Part model, mm, in its own coordinate system. Face numbers are marked on the shaded views. A direction names the side the tool comes from. Coordinates: 2 decimals unless noted, no trailing zeros. Loops run counter-clockwise (first coordinate to the right, second up) from the corner with the lowest first, then second, coordinate; pieces in that order, holes last.
Solid Edge part; units mm, degrees
sketch "Sketch1" plane through (0, 0, 0) normal (0, -1, 0) x (1, 0, 0)
  circle A0 centre (80.5127, 55.3877) radius 22.5
extrude "ExtrudedProtrusion_1" add sketch "Sketch1" against normal blind 10
sketch "Sketch2" plane through (63.9305, 0, 41.9251) normal (0, -1, 0) x (1, 0, 0)
  line L0 (18.5822, 5.9759) -> (18.5822, 0.9759)
  arc A0 (18.5822, 0.9759) -> (14.5822, 0.9759) centre (16.5822, 0.9759) cw
  line L1 (14.5822, 0.9759) -> (14.5822, 5.9759)
  arc A1 (14.5822, 5.9759) -> (9.5822, 10.9759) centre (9.5822, 5.9759) ccw
  line L2 (9.5822, 10.9759) -> (4.5822, 10.9759)
  arc A2 (4.5822, 10.9759) -> (4.5822, 14.9759) centre (4.5822, 12.9759) cw
  line L3 (4.5822, 14.9759) -> (9.5822, 14.9759)
  arc A3 (9.5822, 14.9759) -> (12.5822, 17.9759) centre (9.5822, 17.9759) ccw
  arc A4 (12.5822, 17.9759) -> (20.5822, 17.9759) centre (16.5822, 13.4626) cw
  arc A5 (23.5822, 14.9759) -> (20.5822, 17.9759) centre (23.5822, 17.9759) cw
  line L4 (28.5822, 14.9759) -> (23.5822, 14.9759)
  arc A6 (28.5822, 10.9759) -> (28.5822, 14.9759) centre (28.5822, 12.9759) ccw
  line L5 (23.5822, 10.9759) -> (28.5822, 10.9759)
  arc A7 (18.5822, 5.9759) -> (23.5822, 10.9759) centre (23.5822, 5.9759) cw
  dimension "D1" = 18.5822
  dimension "D2" = 14.5822
  dimension "D3" = 23.5822
  dimension "D4" = 9.5822
  dimension "D5" = 4.5822
  dimension "D6" = 28.5822
extrude "Cutout1" cut sketch "Sketch2" against normal blind 5
sketch "Sketch3" plane through (80.5127, 10, 55.3877) normal (0, 1, 0) x (0, 0, -1)
  circle A0 centre (0, 0) radius 3
extrude "ExtrudedCutout_5" cut sketch "Sketch3" against normal blind 4
sketch "Sketch4" plane through (80.5127, 6, 55.3877) normal (0, 1, 0) x (-1, 0, 0)
  circle A0 centre (0, 0) radius 1.05
extrude "Cutout2" cut sketch "Sketch4" against normal up to next
sketch "Sketch5" plane through (80.5127, 5, 51.1598) normal (0, -1, 0) x (1, 0, 0)
  circle A0 centre (0, 4.2279) radius 3.55
extrude "ExtrudedCutout_7" cut sketch "Sketch5" against normal blind 0.5
chamfer "Chamfer_2" distance 1.9 distance2 0.5 1 edges at (80.5127, 6, 58.3877) measured on face at (78.5727, 6, 53.3277)
sketch "Sketch6" plane through (80.5127, 10, 55.3877) normal (0, 1, 0) x (0, 0, 1)
  circle A0 centre (0, 0) radius 22.5
  circle A1 centre (0, 0) radius 3
extrude "ExtrudedProtrusion_4" add sketch "Sketch6" along normal blind 1.5
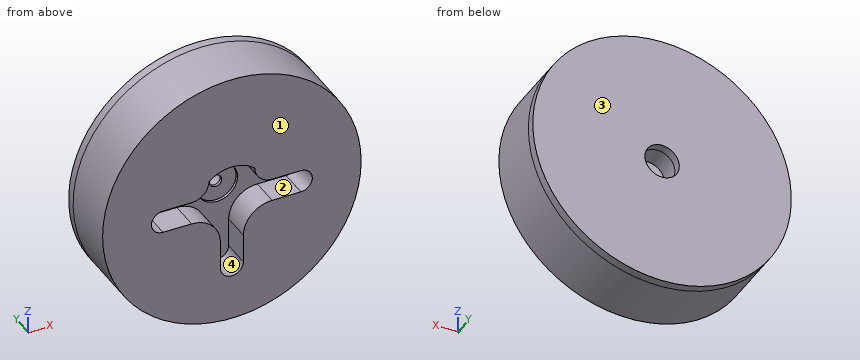
Q1. Probe line 1 (Y direction, x = 67.5, z = 54.5); line 2 (X direction, y = 3.25, z = 60); line 3 (Z direction, x = 79.5, y = 9). List the from-to ranges inside material, lowest first.
Q2. Mould opens along X. For the marked faces 3 and 4 say: released by +X, released by -X, zero draft, split by the parting line, or undercut.
Q3. Saw through at B-B (y = 3). List the corners of the cut face in (x, z).
Q4. Tool access for the marked faces 1 and 2: list every direction of +Z, -Z, +X, -X, +Y, -Y with a clear straight run to the whole face (end or side of a thin tool).
Q5. Drop flat-ended pins along their axis: P1, Ø1.3, axis at x = 80.51, z = 55.39, coming from the -Y side; P2, Ø4.5, axis at x = 80.51, z = 55.39, coming from the -Y side; P3, Ø1.5, axis at x = 71.5, y = 3.5, coming from the -Z side; P4, Ø2.5, axis at x = 91, y = 2.5, coming from the +Z side. Give the stop position or say it passes through.
Q6. Saw through at A-A (x = 89.5). List the corners of the cut face in (y, z).
Q7. Saw through at C-C (z = 44.5). List the corners of the cut face in (x, y), plus the area to 3 significant figures.
Q8. Saw through at D-D (x = 62). List the corners of the cut face in (y, z).
Checked values:
1. line 1: y = 5 to 11.5
1. line 2: x = 58.49 to 76.63, 84.4 to 102.53
1. line 3: z = 32.91 to 52.56, 58.21 to 77.86
2. face 3: zero draft
2. face 4: undercut
3. outline: circle Ø45 at (80.51, 55.39); hole (68.51, 52.9) - (73.51, 52.9) arc R5 cw to (78.51, 47.9) - (78.51, 42.9) arc R2 ccw to (82.51, 42.9) - (82.51, 47.9) arc R5 cw to (87.51, 52.9) - (92.51, 52.9) arc R2 ccw to (92.51, 56.9) - (87.51, 56.9) arc R3 cw to (84.51, 59.9) arc R6.03 ccw to (76.51, 59.9) arc R3 cw to (73.51, 56.9) - (68.51, 56.9) arc R2 ccw to start
4. face 1: +Z, -Z, +X, -X, -Y
4. face 2: -Y
5. P1: passes through
5. P2: stops at y = 5.5
5. P3: stops at z = 34.46
5. P4: stops at z = 75.9
6. outline: (0, 34.76) - (11.5, 34.76) - (11.5, 76.01) - (0, 76.01) - (0, 56.9) - (5, 56.9) - (5, 52.9) - (0, 52.9) - close
7. outline: (60.82, 0) - (78.51, 0) - (78.51, 5) - (82.51, 5) - (82.51, 0) - (100.2, 0) - (100.2, 11.5) - (60.82, 11.5) - close
7. area: 433 mm2
8. outline: (0, 42.6) - (11.5, 42.6) - (11.5, 68.18) - (0, 68.18) - close
